from build123d import *

# Parameters (mm, degrees)
BOSS_EXTRUDE1_DEPTH  = 145
M4_CLEARANCE_HOLE1_D = 4.5
HOLE1_D              = 4.5
HOLE1_DEPTH          = 6


with BuildPart() as part:
    # Sketch1 → Boss-Extrude1 (new body)
    with BuildSketch(Plane(origin=(0, 260, 0), x_dir=(-1, 0, 0), z_dir=(0, -1, 0))):
        Polygon((71.5, -127.5), (61.5, -127.5), (61.5, -97.5), (71.5, -97.5), (71.5, -102.5), (67.5, -102.5), (67.5, -122.5), (71.5, -122.5), align=None)
    extrude(amount=BOSS_EXTRUDE1_DEPTH)

    # M4 Clearance Hole1 (through all)
    with Locations(Plane(origin=(-61.5, 0, 0), x_dir=(0, 0, -1), z_dir=(1, 0, 0))):
        with Locations((-112.5, 247.5), (-112.5, 127.5)):
            Hole(M4_CLEARANCE_HOLE1_D / 2)

    # Hole1
    with Locations(Plane(origin=(-61.5, 0, 0), x_dir=(0, 0, -1), z_dir=(1, 0, 0))):
        with Locations((-104, 216), (-121, 216), (-104, 159), (-121, 159)):
            Hole(HOLE1_D / 2, depth=HOLE1_DEPTH)


solid = part.part
The model under review builds one solid part; all positions refer to its coordinate system, in mm. A direction names the side the tool comes from. Coordinates: 2 decimals unless noted, no trailing zeros. Loops run counter-clockwise (first coordinate to the right, second up) from the corner with the lowest first, then second, coordinate; pieces in that order, holes last. Notation, with made-up numbers: M -40,81 L 5,81 A25 ccw 5,103 Z; hole C 64.25,79 d7. An arc over 180 degrees is marked long. Put each result on its own line as item: value. Start each with the question number.
Q1. Add section A-A (y = 127.5). Write out the cut boundary in (x, z), and give its area (3 significant figures).
Q2. Clearance check with flat-ended pins moving along their axes: pin 1 (6 mm diameter, centred on y = 127.5, z = 112.5, fed in from -X); pin 2 (3.5 mm diameter, centred on y = 159, z = 104, fed in from +X). State where each tip first meets the part, or that it passes through.
Q3. Add section D-D (y = 216). Write out the cut boundary in (x, z), and give its area (3 significant figures).
Q4. For faces 5 (the flat face through (-66, 189, 97.5)), 6 (the flat face through (-69, 189, 122.5)), 7 (the cylindrical face through (-64.54, 158.14, 106.08)), list the 3-axis set-ups (+Z, -Z, +X, -X, +Y, -Y) from which the entire face can be reached by the end or side of a thin tool; tool diameter is ignored.
Q5. Wall thickness on line 1 (Y direction, x = -65.3, z = 104); line 2 (Z direction, x = -64.35, y = 159); line 3 (Y direction, x = -66.15, z = 112.5): over which ranges is each line inside the solid? List them lowest first.
Q6. Add section C-C (z = 104). Write out the cut boundary in (x, y).
Q7. Add section B-B (x = -66). Write out the cut boundary in (y, z), and give its area (3 significant figures).
Q8. The part is to be moulded in two halves that separate along Y. For faces 1 (the flat face through (-71.5, 189, 125)), 2 (the flat face through (-65, 260, 112)), 3 (the cylindrical face through (-64.542, 249.397, 113.71)), 4 (the flat face through (-65, 115, 112)), say which applies: +Y half, -Y half, draft (parallel to the pull), parting line (faces both ways), or undercut.
Answers:
1. outline: M -71.5,97.5 L -61.5,97.5 L -61.5,110.25 L -67.5,110.25 L -67.5,102.5 L -71.5,102.5 Z; M -71.5,122.5 L -67.5,122.5 L -67.5,114.75 L -61.5,114.75 L -61.5,127.5 L -71.5,127.5 Z
1. area: 193 mm^2
2. pin 1: stops at x = -67.5
2. pin 2: stops at x = -67.5
3. outline: M -71.5,97.5 L -61.5,97.5 L -61.5,101.75 L -67.5,101.75 L -67.5,102.5 L -71.5,102.5 Z; M -71.5,122.5 L -67.5,122.5 L -67.5,123.25 L -61.5,123.25 L -61.5,127.5 L -71.5,127.5 Z; M -67.5,106.25 L -61.5,106.25 L -61.5,118.75 L -67.5,118.75 Z
3. area: 166 mm^2
4. face 5: -Z, +X, -X, +Y, -Y
4. face 6: -X, +Y, -Y
4. face 7: +X
5. line 1: y = 115 to 156.75, 161.25 to 213.75, 218.25 to 260
5. line 2: z = 97.5 to 101.75, 106.25 to 118.75, 123.25 to 127.5
5. line 3: y = 115 to 125.25, 129.75 to 245.25, 249.75 to 260
6. outline: M -67.5,115 L -61.5,115 L -61.5,156.75 L -67.5,156.75 Z; M -67.5,161.25 L -61.5,161.25 L -61.5,213.75 L -67.5,213.75 Z; M -67.5,218.25 L -61.5,218.25 L -61.5,260 L -67.5,260 Z
7. outline: M 115,97.5 L 260,97.5 L 260,127.5 L 115,127.5 Z; hole C 127.5,112.5 d4.5; hole C 159,104 d4.5; hole C 159,121 d4.5; hole C 216,104 d4.5; hole C 216,121 d4.5; hole C 247.5,112.5 d4.5
7. area: 4,250 mm^2
8. face 1: draft
8. face 2: +Y half
8. face 3: undercut
8. face 4: -Y half
